Design review of the part built by this model. Coordinates are the model's own, in mm. A direction names the side the tool comes from. Give positions to 0.01 mm unless a question says otherwise; leave off trailing zeros. Order: outer loops, then holes, each group sorted by start corner. A loop starts at its lowest first (then second) coordinate and runs counter-clockwise, first axis right, second up. Notation, with made-up numbers: (40.25, 10.25) -> (56.25, 10.25) arc R22 cw to (56.25, 38.25) -> close; hole circle Ø7 at (48.25, 83.25). An arc over 180 degrees is marked (long way). Return JSON: item names as keys, results as strings.
Autodesk Inventor part; units mm, degrees
ref_plane "YZ Plane" through (0, 0, 0) normal (1, 0, 0) x (0, 1, 0)
ref_plane "XZ Plane" through (0, 0, 0) normal (0, 1, 0) x (-1, 0, 0)
ref_plane "XY Plane" through (0, 0, 0) normal (0, 0, 1) x (1, 0, 0)
sketch "Sketch1" plane through (0, 0, 0) normal (1, 0, 0) x (0, 1, 0)
  line L0 (7.3323, 0) -> (3.6662, -6.35)
  line L1 (3.6662, -6.35) -> (-3.6662, -6.35)
  line L2 (-3.6662, -6.35) -> (-7.3323, 0)
  line L3 (-7.3323, 0) -> (-3.6662, 6.35)
  line L4 (-3.6662, 6.35) -> (3.6662, 6.35)
  line L5 (3.6662, 6.35) -> (7.3323, 0)
  circle A0 centre (0, 0) radius 6.35
  dimension "d0" = 12.7
extrude "Extrusion1" add sketch "Sketch1" along normal blind 22.844
extrude "Extrusion2" add sketch "Sketch1" against normal blind 7.9248 contours A0
ref_plane "Work Plane1" through (0, 7.3323, 0) normal (0, 0, -1) x (1, 0, 0)
sketch "Sketch2" plane through (0, 7.3323, 0) normal (0, 0, -1) x (1, 0, 0)
  line L0 (0, 13.6823) -> (-7.9248, 13.6823)
  line L1 (0, 10.9985) -> (0, 14.6647)
  line L2 (0, 14.6647) -> (22.844, 14.6647)
  line L3 (11.8966, 14.6647) -> (12.684, 14.6647)
  line L4 (12.684, 14.6647) -> (12.684, 13.6823)
  line L5 (12.684, 13.6823) -> (11.8966, 13.6823)
  line L6 (11.8966, 13.6823) -> (11.8966, 14.6647)
  line L7 (0, 7.3323) -> (22.844, 7.3323)
  line L8 (22.844, 3.6662) -> (22.844, 10.9985)
  line L9 (22.844, 14.6647) -> (22.844, 10.9985)
  dimension "d7" = 0.7874
  dimension "d9" = 10.16
revolve "Revolution1" cut sketch "Sketch2" angle 360 about axis through (0, 0, 0) along (1, 0, 0)
sketch "Sketch3" plane through (22.844, 0, 0) normal (1, 0, 0) x (0, 0, -1)
  line L0 (6.35, 3.6662) -> (0, 7.3323)
  line L1 (0, 7.3323) -> (-6.35, 3.6662)
  line L2 (-6.35, 3.6662) -> (-6.35, -3.6662)
  line L3 (-6.35, -3.6662) -> (0, -7.3323)
  line L4 (0, -7.3323) -> (6.35, -3.6662)
  line L5 (6.35, -3.6662) -> (6.35, 3.6662)
  point P0 (0, 0)
extrude "Extrusion3" add sketch "Sketch3" along normal blind 100
properties part number "LongShaft"
Item 1: Mouldability with a two-part tool opening along X and no side actions: class faces 5 (the face through (0, -3, 6)), 6 (the face through (12.684, -3, 6)), 7 (the face through (67, 0, 6.35)) as released by +X, released by -X, zero draft, split by the parting line, or undercut.
Result set:
{"face 5": "released by -X", "face 6": "undercut", "face 7": "zero draft"}
Item 2: Wall thickness on L1, parallel to Z at x = 62, y = -4.25; L2, parallel to Y at x = 44.5, z = 0.5; L3, parallel to Y at x = 57, z = 5.25: over which ranges is each line inside the solid? List them lowest first. Write a range as [from, to].
Result set:
{"L1": "z = [-5.34, 5.34]", "L2": "y = [-7.04, 7.04]", "L3": "y = [-4.3, 4.3]"}
Item 3: Machinability: for faces 1 (the face through (12.684, -3, -6)), 2 (the face through (12.28, 1.38, -6.2)), 3 (the face through (11.897, -3, 6)), 4 (the face through (12.684, 3, -6)), which of the approach directions +Z, -Z, +X, -X, +Y, -Y give a long, thin tool a straight path to every point of the face, cutting with its end or side? Answer none if there is none.
Result set:
{"face 1": "-Z, -Y", "face 2": "none", "face 3": "+Z, -Y", "face 4": "-Z, +Y"}
Item 4: For pin 1 (3 mm diameter, centred on x = 57, z = 2.5, fed in from +Y); pin 2 (1.5 mm diameter, centred on y = 6.5, z = 1, fed in from -X), all flat-tipped, find the tip position at first contact; note any pin that passes through.
Result set:
{"pin 1": "stops at y = 6.75", "pin 2": "stops at x = -7.92"}
Item 5: Add section A-A (x = 36.5). Give the boundary of the cut face in (y, z), plus the area to 3 significant figures.
Result set:
{"outline": "(-7.33, 0) -> (-3.67, -6.35) -> (3.67, -6.35) -> (7.33, 0) -> (3.67, 6.35) -> (-3.67, 6.35) -> close", "area": "140 mm^2"}
